Geometry check sheet. Reference: drawing and pictorial views, mm from the part's lowest x, y, z. A direction names the side the tool comes from. Coordinates: 2 decimals unless noted, no trailing zeros. Loops run counter-clockwise (first coordinate to the right, second up) from the corner with the lowest first, then second, coordinate; pieces in that order, holes last. Notation, with made-up numbers: (14.5, 2.5) -> (36.5, 2.5) arc R18 ccw to (36.5, 14.5) -> close; hole circle Ø10 at (40, 59.25). An arc over 180 degrees is marked (long way). Answer as a JSON object with one key per item and string values.
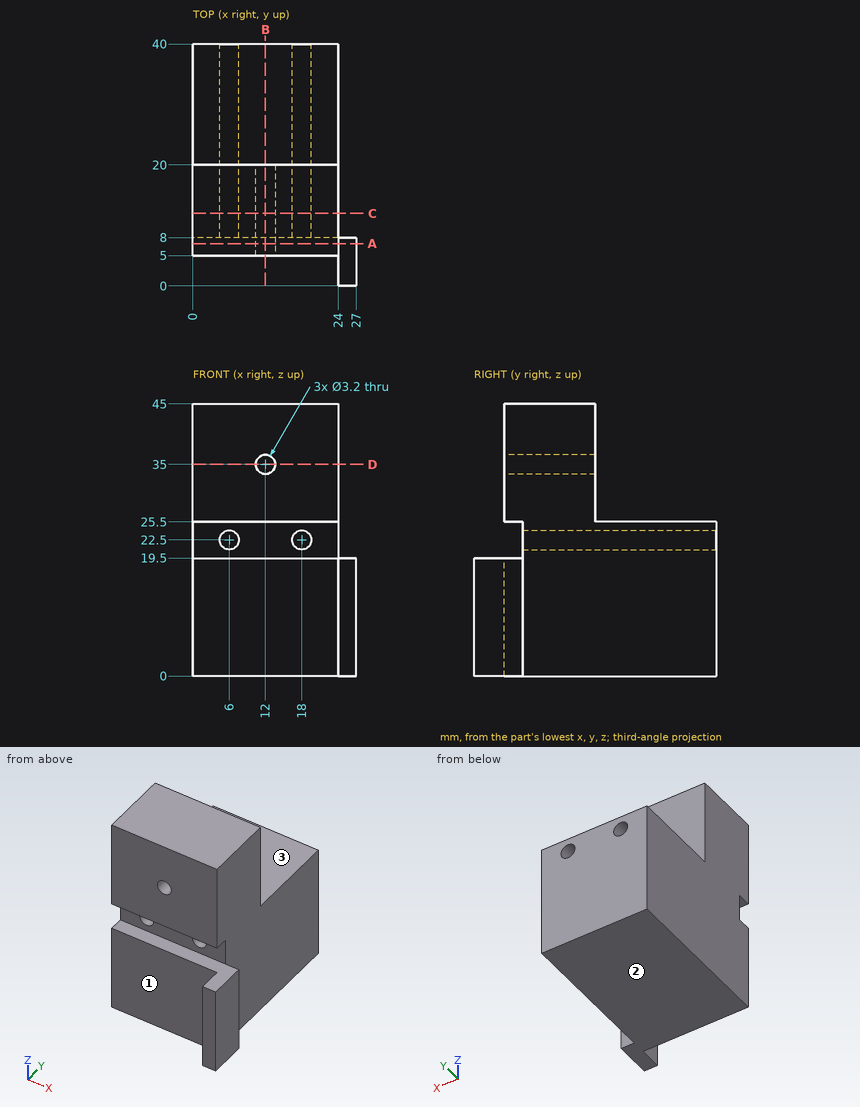
1. Section check B-B, the plane x = 12. Record the boundary of the cut face in (y, z).
Evaluation:
{"outline": "(5, 0) -> (40, 0) -> (40, 25.5) -> (20, 25.5) -> (20, 33.4) -> (5, 33.4) -> (5, 25.5) -> (8, 25.5) -> (8, 19.5) -> (5, 19.5) -> close; (5, 36.6) -> (20, 36.6) -> (20, 45) -> (5, 45) -> close"}
2. Depth check by flat-ended pin: P1, Ø1, axis at y = 21.5, z = 9.5, coming from the +X side; P2, Ø15.5, axis at x = 6, z = 33, coming from the -Y side; P3, Ø10, axis at x = 14.5, z = 37, coming from the +Y side. Enter the tip coordinate at first touch or a pass-through.
Evaluation:
{"P1": "stops at x = 24", "P2": "stops at y = 5", "P3": "stops at y = 20"}
3. Section check A-A, the plane y = 7. Record the boundary of the cut face in (x, z).
Evaluation:
{"outline": "(0, 0) -> (27, 0) -> (27, 19.5) -> (0, 19.5) -> close; (0, 25.5) -> (24, 25.5) -> (24, 45) -> (0, 45) -> close; hole circle Ø3.2 at (12, 35)"}
4. Section check D-D, the plane z = 35. Record the boundary of the cut face in (x, y).
Evaluation:
{"outline": "(0, 5) -> (10.4, 5) -> (10.4, 20) -> (0, 20) -> close; (13.6, 5) -> (24, 5) -> (24, 20) -> (13.6, 20) -> close"}
5. Thickness scan on probe 1 along X at (y, z) = (15.5, 35); probe 2 along X at (y, z) = (17, 22); probe 3 along Z at (x, y) = (3.25, 7.5). Record the ranges inside material, lowest first. Write a range as from..to.
Evaluation:
{"probe 1": "x = 0..10.4, 13.6..24", "probe 2": "x = 0..4.48, 7.52..16.48, 19.52..24", "probe 3": "z = 0..19.5, 25.5..45"}
6. Tool access check on the marked faces 1, 2 and 3. Record the directions out of +Z, -Z, +X, -X, +Y, -Y that give a thin tool (end or side, any length) a straight path to the whole face; none if there is none.
Evaluation:
{"face 1": "+Z, -Z, -X, -Y", "face 2": "-Z, +X, -X, +Y, -Y", "face 3": "+Z, +X, -X, +Y"}
7. Section check C-C, the plane y = 12. Record the boundary of the cut face in (x, z).
Evaluation:
{"outline": "(0, 0) -> (24, 0) -> (24, 45) -> (0, 45) -> close; hole circle Ø3.2 at (6, 22.5); hole circle Ø3.2 at (12, 35); hole circle Ø3.2 at (18, 22.5)"}
